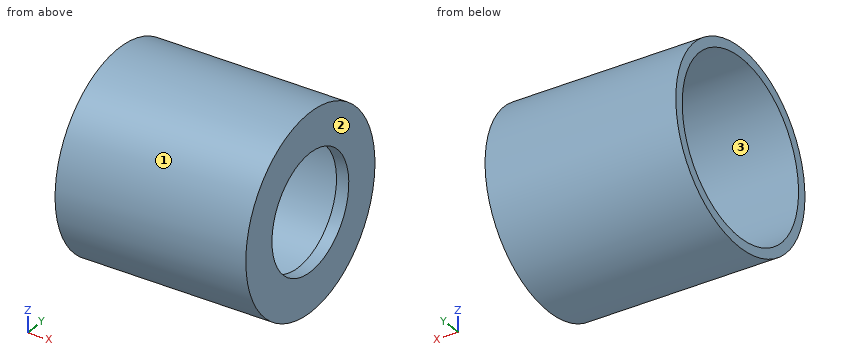
```python
from build123d import *

# Parameters (mm, degrees)
SKETCH1_R          = 4.0005
EXTRUDE1_DEPTH     = 7.874
SKETCH2_R          = 3.603625
CUT_EXTRUDE1_DEPTH = 7.366
SKETCH3_R          = 2.38125
CUT_EXTRUDE2_DEPTH = 1.508


with BuildPart() as part:
    # Sketch1 → Extrude1 (new body)
    with BuildSketch(Plane(origin=(0, 0, 0), x_dir=(0, 0, -1), z_dir=(1, 0, 0))):
        Circle(SKETCH1_R)
    extrude(amount=EXTRUDE1_DEPTH)

    # Sketch2 → Cut-Extrude1 (cut)
    with BuildSketch(Plane.ZY):
        Circle(SKETCH2_R)
    extrude(amount=-CUT_EXTRUDE1_DEPTH, mode=Mode.SUBTRACT)

    # Sketch3 → Cut-Extrude2 (cut, through all)
    with BuildSketch(Plane.ZY.offset(-7.366)):
        Circle(SKETCH3_R)
    extrude(amount=-CUT_EXTRUDE2_DEPTH, mode=Mode.SUBTRACT)


solid = part.part
```
Here's how the part is built. I have some questions about the finished solid (model axes, mm). Face numbers are marked on the shaded views. Coordinates: 2 decimals unless noted, no trailing zeros. Write each loop counter-clockwise with the first axis right and the second up, starting at its lowest first coordinate (ties: lowest second). Pieces come first, ordered by that corner, then holes. Notation, with made-up numbers: (-21.75, 9) -> (-12.75, 9) arc R24 cw to (-12.75, 32) -> close; hole circle Ø7 at (-33, 41.5). An arc over 180 degrees is marked (long way). Use a Markdown table: item, result. Add a question column.
(1) If we section it at A-A, the plane z = 0: Write out the boundary of the cut face in (x, y).
(2) If we section it at D-D, the plane y = -2.75: Write out the boundary of the cut face in (x, z).
(3) If we section it at C-C, the plane x = 6.75: Write out the boundary of the cut face in (y, z).
(4) Please list where these lines run through material, in increasing order: line 1 (Y direction, x = 3.25, z = 0); line 2 (Y direction, x = 3.5, z = -1.5).
(5) We'd pull the mould along Y, two halves only. Please class the marked faces 1, 2 and 3: +Y half, -Y half, draft (parallel to the pull), parting line (faces both ways), or undercut.
(6) I'm going to push flat-ended pins straight in: P1, Ø3, axis at y = 0, z = 0, coming from the +X side; P2, Ø2, axis at y = -0.5, z = -2, coming from the -X side; P3, Ø1, axis at x = 4, y = 2, coming from the +Z side; P4, Ø2, axis at x = 2.5, z = -3, coming from the -Y side. Where does each tip first touch, or does it pass through?
Outcome:
| question | item | result |
|---|---|---|
| 1 | outline | (0, -4) -> (7.87, -4) -> (7.87, -2.38) -> (7.37, -2.38) -> (7.37, -3.6) -> (0, -3.6) -> close; (0, 3.6) -> (7.37, 3.6) -> (7.37, 2.38) -> (7.87, 2.38) -> (7.87, 4) -> (0, 4) -> close |
| 2 | outline | (0, -2.91) -> (7.87, -2.91) -> (7.87, 2.91) -> (0, 2.91) -> (0, 2.33) -> (7.37, 2.33) -> (7.37, -2.33) -> (0, -2.33) -> close |
| 3 | outline | circle Ø8 at (0, 0); hole circle Ø7.21 at (0, 0) |
| 4 | line 1 | y = -4 to -3.6, 3.6 to 4 |
| 4 | line 2 | y = -3.71 to -3.28, 3.28 to 3.71 |
| 5 | face 1 | parting line |
| 5 | face 2 | draft |
| 5 | face 3 | undercut |
| 6 | P1 | passes through |
| 6 | P2 | stops at x = 7.37 |
| 6 | P3 | stops at z = 3.71 |
| 6 | P4 | stops at y = -3.46 |
